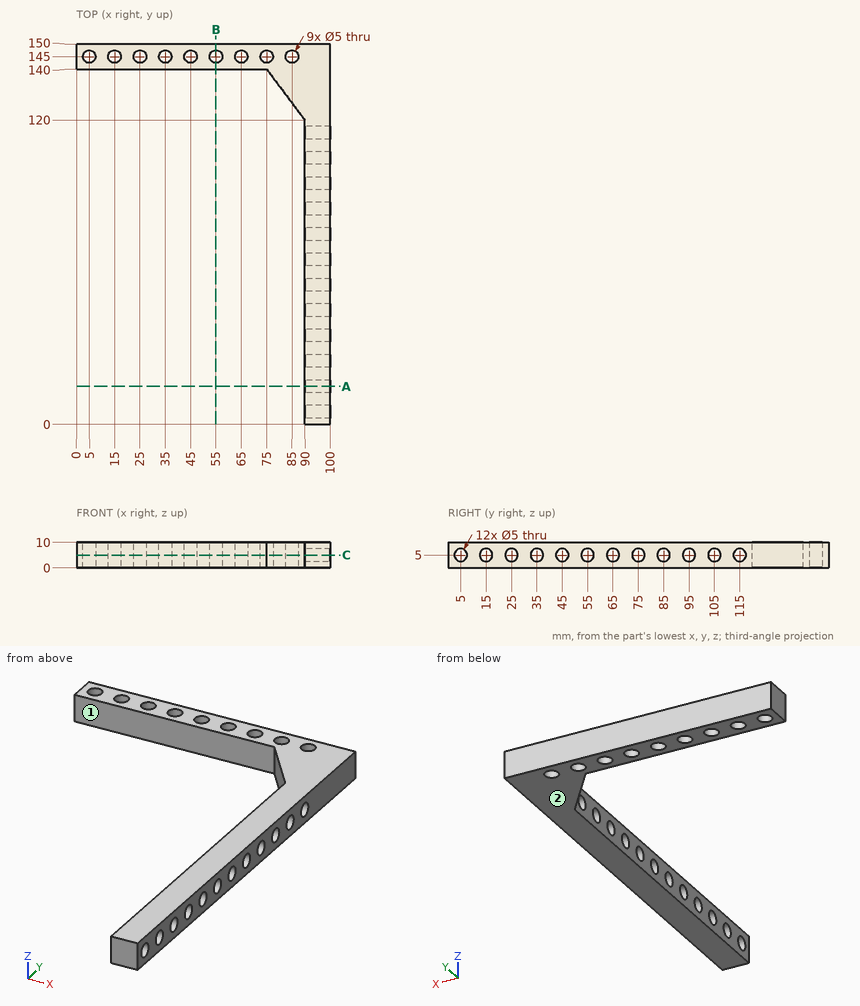
The figure shows three views and two pictorial views of one solid part (mm, origin at its lowest corner). Answer the questions. A direction names the side the tool comes from. Coordinates: 2 decimals unless noted, no trailing zeros. Loops run counter-clockwise (first coordinate to the right, second up) from the corner with the lowest first, then second, coordinate; pieces in that order, holes last. Notation, with made-up numbers: (9.5, 8) -> (55.5, 8) arc R13 cw to (55.5, 19) -> close; hole circle Ø5 at (88, 10). An arc over 180 degrees is marked (long way). Write item = value, one per line. Start each with the question number.
1) A cutting plane is placed at C-C (z = 5). Count the separate pieces of the cut face and the enclosed holes in it, then the cut area to 3 significant figures.
2) A tool of negligible diameter and unlimited length cuts with its end or side. For the marked faces 1 and 2, from which of +Z, -Z, +X, -X, +Y, -Y can it reach the whole face along a straight path? Write none if from no direction.
3) Given pin 1 Ø6 at (y, z) = (15, 5) entering from -X; pin 2 Ø3 at (x, y) = (45, 145) entering from -Z; pin 3 Ø2 at (x, z) = (23, 9) entering from -Y, each flat-ended and moving along its own axis, determine where each tip first touches the part or whether it passes through.
4) A cutting plane is placed at B-B (x = 55). Give the vertices of the cut face in (y, z).
5) A cutting plane is placed at A-A (y = 15). Give the vertices of the cut face in (x, z).
6) Straight lines are drawn through the part: line 1 (Y direction, x = 35, z = 6.5); line 2 (Z direction, x = 97, y = 5); line 3 (Y direction, x = 41, z = 6.5). For each, find the intervals that lie inside material, in ascending order. Write a range as from..to.
Responses:
q1.separate_pieces = 13
q1.enclosed_holes = 9
q1.area = 1,770 mm²
q2.face_1 = +Z, -Z, -X, -Y
q2.face_2 = -Z, +X, -X, +Y, -Y
q3.pin_1 = 90
q3.pin_2 = through
q3.pin_3 = 140
q4.outline = (140, 0) -> (142.5, 0) -> (142.5, 10) -> (140, 10) -> close; (147.5, 0) -> (150, 0) -> (150, 10) -> (147.5, 10) -> close
q5.outline = (90, 0) -> (100, 0) -> (100, 2.5) -> (90, 2.5) -> close; (90, 7.5) -> (100, 7.5) -> (100, 10) -> (90, 10) -> close
q6.line_1 = 140..142.5, 147.5..150
q6.line_2 = 0..2.5, 7.5..10
q6.line_3 = 140..150
